CAD build for the part. Positions are in the model's coordinates, mm. Round coordinates to 2 decimals unless told otherwise and drop trailing zeros. Loops run counter-clockwise (first coordinate to the right, second up) from the corner with the lowest first, then second, coordinate; pieces in that order, holes last.
```python
from build123d import *

# Parameters (mm, degrees)
SKETCH1_W           = 84.5
SKETCH1_H           = 250
BOSS_EXTRUDE1_DEPTH = 5
SKETCH2_W           = 84.5
SKETCH2_H           = 5
BOSS_EXTRUDE2_DEPTH = 25.4
SKETCH3_R           = 4.7625
BOSS_EXTRUDE3_DEPTH = 20


with BuildPart() as part:
    # Sketch1 → Boss-Extrude1 (new body)
    with BuildSketch(Plane.XY):
        Rectangle(SKETCH1_W, SKETCH1_H)
    extrude(amount=BOSS_EXTRUDE1_DEPTH)

    # Sketch2 → Boss-Extrude2 (add)
    with BuildSketch(Plane.XY.offset(5)):
        with Locations((0, -122.5)):
            Rectangle(SKETCH2_W, SKETCH2_H)
    extrude(amount=BOSS_EXTRUDE2_DEPTH)

    # Sketch3 → Boss-Extrude3 (add)
    with BuildSketch(Plane.XY.offset(5)):
        with Locations((2.625, 10)):
            Circle(SKETCH3_R)
    extrude(amount=BOSS_EXTRUDE3_DEPTH)


solid = part.part
```
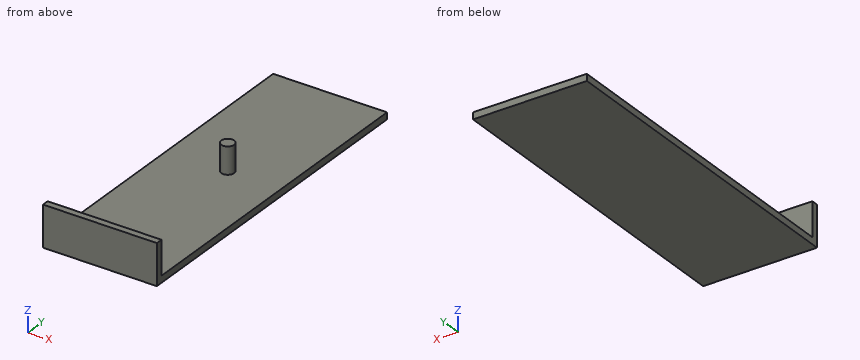
Item 1: Probe line 1 (Z direction, x = 24.5, y = 70); line 2 (Y direction, x = 25, z = 9); line 3 (X direction, y = 7, z = 13). List the from-to ranges inside material, lowest first.
Answers follow:
line 1: z = 0 to 5
line 2: y = -125 to -120
line 3: x = -1.07 to 6.32
Item 2: Cut at C-C, the plane x = -11. Give the cut face in (y, z).
Answers follow:
outline: (-125, 0) - (125, 0) - (125, 5) - (-120, 5) - (-120, 30.4) - (-125, 30.4) - close
Item 3: Cut at B-B, the plane y = 10. Give the cut face in (x, z).
Answers follow:
outline: (-42.25, 0) - (42.25, 0) - (42.25, 5) - (7.39, 5) - (7.39, 25) - (-2.14, 25) - (-2.14, 5) - (-42.25, 5) - close
Item 4: Flat gauge pins, fed straight in: P1, Ø5, axis at x = 1.5, y = 12, coming from the +Z side; P2, Ø1.5, axis at x = 32.5, z = 26.5, coming from the +Y side. Where does each tip first touch, or does it go through?
Answers follow:
P1: stops at z = 25
P2: stops at y = -120
Item 5: Cut at D-D, the plane z = 28. Give the cut face in (x, y), plus the area to 4 significant figures.
Answers follow:
outline: (-42.25, -125) - (42.25, -125) - (42.25, -120) - (-42.25, -120) - close
area: 422.5 mm2
